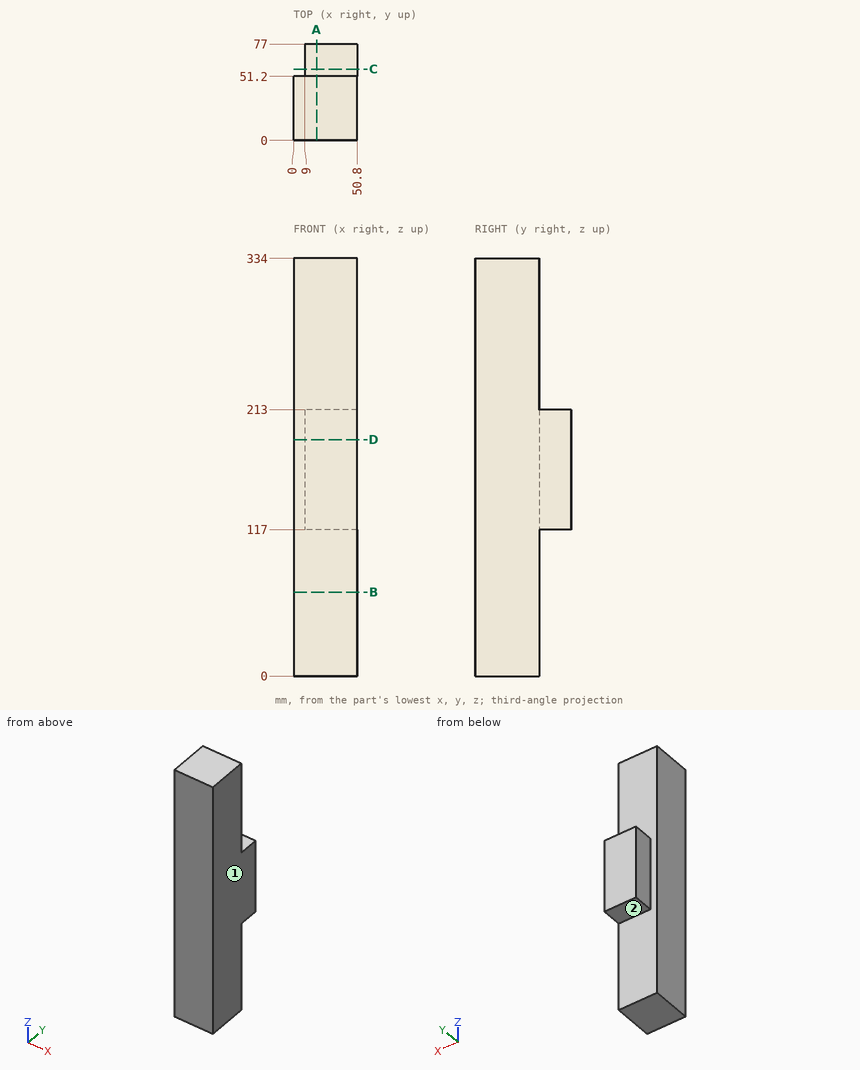
Design review of the part shown in the three views and the two pictorial views. Dimensions are in mm from the part's minimum x, y and z. A direction names the side the tool comes from. Give positions to 0.01 mm unless a question says otherwise; leave off trailing zeros. Loops run counter-clockwise (first coordinate to the right, second up) from the corner with the lowest first, then second, coordinate; pieces in that order, holes last. Notation, with made-up numbers: (30.5, 26.5) -> (81.5, 26.5) arc R25 cw to (81.5, 62.5) -> close; hole circle Ø4 at (60.5, 16.25). An arc over 180 degrees is marked (long way). One line per question, with ' | ' between items.
1) Insertion check: pin 1 Ø7.5 at (x, y) = (37, 58) entering from -Z; pin 2 Ø3 at (x, z) = (5.5, 149) entering from -Y; pin 3 Ø7.5 at (x, y) = (30, 67.5) entering from +Z. Each pin has a flat end and moves straight along its axis. Give the tip position at first contact, or say it passes through.
Resolved:
pin 1: stops at z = 117 | pin 2: stops at y = 0 | pin 3: stops at z = 213
2) We need section A-A (x = 18.5). Write out the cut boundary in (y, z), plus the area to 3 significant figures.
Resolved:
outline: (0, 0) -> (51.2, 0) -> (51.2, 117) -> (77, 117) -> (77, 213) -> (51.2, 213) -> (51.2, 334) -> (0, 334) -> close | area: 19,600 mm2
3) For the marked faces 1 and 2, list the 3-axis set-ups (+Z, -Z, +X, -X, +Y, -Y) from which the entire face can be reached by the end or side of a thin tool; tool diameter is ignored.
Resolved:
face 1: +Z, -Z, +X, +Y, -Y | face 2: -Z, +X, -X, +Y
4) We need section B-B (z = 67). Write out the cut boundary in (x, y).
Resolved:
outline: (0, 0) -> (50.8, 0) -> (50.8, 51.2) -> (0, 51.2) -> close
5) We need section D-D (z = 189). Write out the cut boundary in (x, y).
Resolved:
outline: (0, 0) -> (50.8, 0) -> (50.8, 77) -> (9, 77) -> (9, 51.2) -> (0, 51.2) -> close
6) We need section C-C (y = 57). Write out the cut boundary in (x, z), plus the area to 3 significant figures.
Resolved:
outline: (9, 117) -> (50.8, 117) -> (50.8, 213) -> (9, 213) -> close | area: 4,010 mm2
7) To check wall thickness, follow probe 1 along Y at (x, z) = (42, 303.5); probe 2 along Z at (x, y) = (13.5, 53); probe 3 along X at (y, z) = (57, 167.5). State the ranges of each line that lie inside material, in increasing order.
Resolved:
probe 1: y = 0 to 51.2 | probe 2: z = 117 to 213 | probe 3: x = 9 to 50.8
